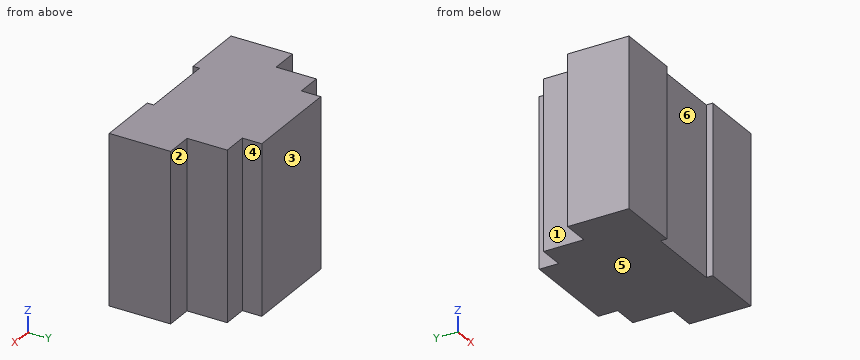
Autodesk Inventor part; units mm, degrees
ref_plane "YZ Plane" through (0, 0, 0) normal (1, 0, 0) x (0, 1, 0)
ref_plane "XZ Plane" through (0, 0, 0) normal (0, 1, 0) x (-1, 0, 0)
ref_plane "XY Plane" through (0, 0, 0) normal (0, 0, 1) x (1, 0, 0)
sketch "Sketch1" plane through (0, 0, 0) normal (0, 1, 0) x (-1, 0, 0)
  line L0 (0, 0) -> (93, 0)
  line L1 (93, 0) -> (93, -78)
  line L2 (93, -78) -> (0, -78)
  line L3 (0, -78) -> (0, 0)
  dimension "d0" = 78
  dimension "d1" = 93
extrude "Extrusion1" add sketch "Sketch1" along normal blind 56
sketch "Sketch2" plane through (0, 0, 0) normal (0, -1, 0) x (1, 0, 0)
  line L0 (-93, 0) -> (0, 0)
  line L1 (0, -78) -> (-93, -78)
  line L2 (-29, 0) -> (-64, 0)
  line L3 (-64, 0) -> (-64, -78)
  line L4 (-64, -78) -> (-29, -78)
  line L5 (-29, -78) -> (-29, 0)
  line L6 (-93, -78) -> (-93, 0)
  dimension "d4" = 29
  dimension "d5" = 35
extrude "Extrusion2" cut sketch "Sketch2" against normal blind 3 contours L0 L5 L1 L3
sketch "Sketch3" plane through (0, 56, 0) normal (0, 1, 0) x (1, 0, 0)
  line L0 (0, 78) -> (-29, 78)
  line L1 (0, 0) -> (-12.5, 0)
  line L2 (-12.5, 0) -> (-12.5, 78)
  line L3 (-12.5, 78) -> (0, 78)
  line L4 (0, 78) -> (0, 0)
  line L5 (-93, 0) -> (-64, 0)
  line L6 (-93, 0) -> (-80.5, 0)
  line L7 (-80.5, 0) -> (-80.5, 78)
  line L8 (-80.5, 78) -> (-93, 78)
  line L9 (-93, 78) -> (-93, 0)
  dimension "d8" = 12.5
  dimension "d9" = 12.5
extrude "Extrusion3" cut sketch "Sketch3" against normal blind 27.6
sketch "Sketch4" plane through (0, 56, 0) normal (0, 1, 0) x (1, 0, 0)
  line L0 (-80.5, 0) -> (-12.5, 0)
  line L1 (-12.5, 78) -> (-80.5, 78)
  line L2 (-12.5, 0) -> (-24, 0)
  line L3 (-24, 0) -> (-24, 78)
  line L4 (-24, 78) -> (-12.5, 78)
  line L5 (-12.5, 78) -> (-12.5, 0)
  line L6 (-80.5, 0) -> (-69, 0)
  line L7 (-69, 0) -> (-69, 78)
  line L8 (-69, 78) -> (-80.5, 78)
  line L9 (-80.5, 78) -> (-80.5, 0)
  point P0 (0, 0)
  dimension "d12" = 11.5
  dimension "d13" = 11.5
extrude "Extrusion4" cut sketch "Sketch4" against normal blind 9 contours L9 L1 L7 L0 | L3 L1 L5 L0
properties part number "Supply"
Can you work these out from the model? Positions are in its coordinate system, mm. Face numbers are marked on the shaded views. A direction names the side the tool comes from. Round coordinates to 2 decimals unless told otherwise and drop trailing zeros. Write each loop counter-clockwise with the first axis right and the second up, starting at its lowest first coordinate (ties: lowest second). Pieces come first, ordered by that corner, then holes. Notation, with made-up numbers: M -14,65 L 43,65 A16 cw 43,74 Z; hole C 38,80.5 d9. An arc over 180 degrees is marked long. Use a Markdown table: item, result.
Item 1: I want a section at A-A (z = -40.5). List the corners of the cut face in (x, y) for me.
Found:
| item | result |
|---|---|
| outline | M -93,0 L -64,0 L -64,3 L -29,3 L -29,0 L 0,0 L 0,28.4 L -12.5,28.4 L -12.5,47 L -24,47 L -24,56 L -69,56 L -69,47 L -80.5,47 L -80.5,28.4 L -93,28.4 Z |
Item 2: If I drill on line 1 along X through (y, z) = (30.5, -49.5); line 2 along Y through (x, z) = (-56, -38.5); line 3 along Y through (x, z) = (-73.5, -62), over which ranges is the centre line in solid material (lowest first)? Write a range as [from, to].
Found:
| item | result |
|---|---|
| line 1 | x = [-80.5, -12.5] |
| line 2 | y = [3, 56] |
| line 3 | y = [0, 47] |
Item 3: For pin 1 Ø2 at (x, z) = (-11, -61.5) entering from +Y; pin 2 Ø6 at (x, y) = (-75, 11.5) entering from +Z; pin 3 Ø10 at (x, z) = (-8, -33.5) entering from +Y; pin 4 Ø9.5 at (y, z) = (33.5, -56.5) entering from -X, each with a flat end and sliding along its axis, tell me the tip position at first contact or that it passes through.
Found:
| item | result |
|---|---|
| pin 1 | stops at y = 28.4 |
| pin 2 | stops at z = 0 |
| pin 3 | stops at y = 47 |
| pin 4 | stops at x = -80.5 |
Item 4: I want a section at C-C (y = 52). List the corners of the cut face in (x, z) for me, and give its area (3 significant figures).
Found:
| item | result |
|---|---|
| outline | M -69,-78 L -24,-78 L -24,0 L -69,0 Z |
| area | 3,510 mm2 |
Item 5: We'd pull the mould along X, two halves only. Please class the marked faces 4, 5 and 6: released by +X, released by -X, zero draft, split by the parting line, or undercut.
Found:
| item | result |
|---|---|
| face 4 | released by +X |
| face 5 | zero draft |
| face 6 | undercut |
Item 6: I want a section at B-B (x = -56.5). List the corners of the cut face in (y, z) for me, and give its area (3 significant figures).
Found:
| item | result |
|---|---|
| outline | M 3,-78 L 56,-78 L 56,0 L 3,0 Z |
| area | 4,130 mm2 |
Item 7: Which directions (+Z, -Z, +X, -X, +Y, -Y) give clear straight access to the entire face, cutting with the end or side of a thin tool? Please do the marked faces 1, 2 and 3.
Found:
| item | result |
|---|---|
| face 1 | +Z, -Z, -X, +Y |
| face 2 | +Z, -Z, +X, +Y |
| face 3 | +Z, -Z, +X, -X, +Y |
